Geometry check sheet. Reference: drawing and pictorial views, mm from the part's lowest x, y, z. Give positions to 0.01 mm unless a question says otherwise; leave off trailing zeros. Write each loop counter-clockwise with the first axis right and the second up, starting at its lowest first coordinate (ties: lowest second). Pieces come first, ordered by that corner, then holes.
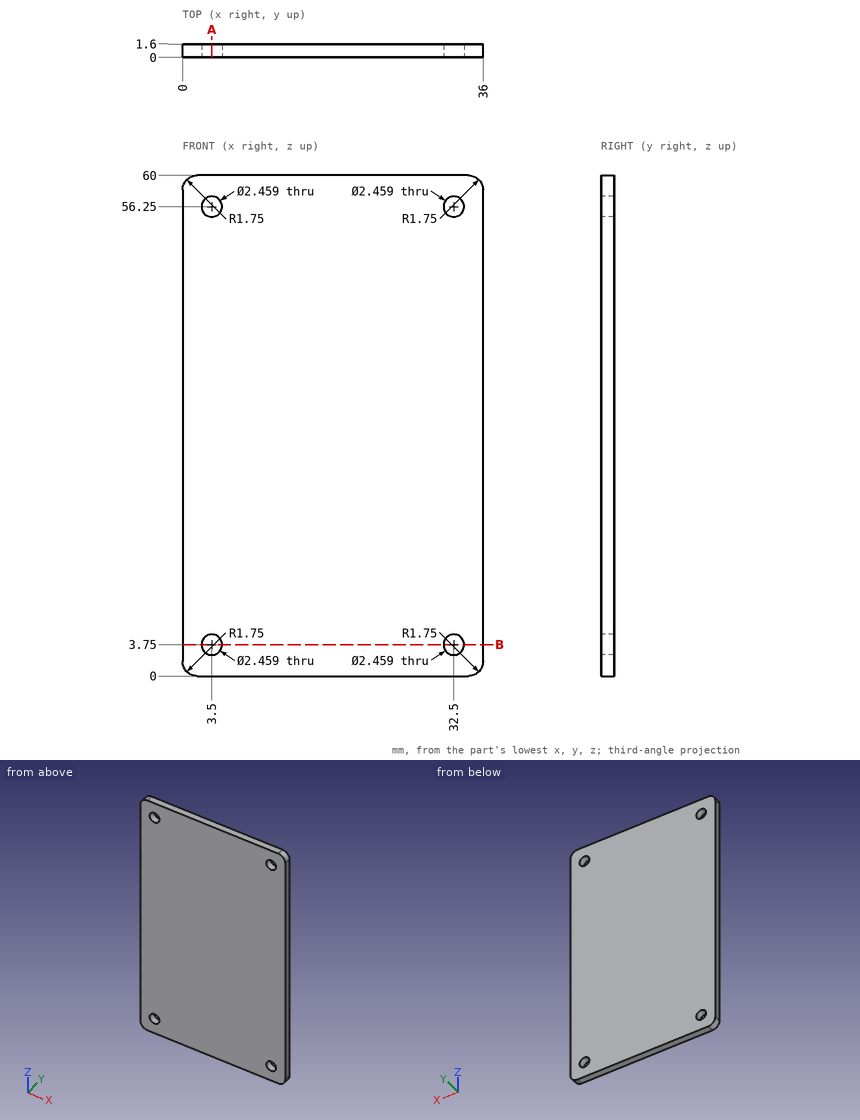
Item 1: Scan lines: line 1 along Z through (x, y) = (32.5, 1.2); line 2 along X through (y, z) = (0.3, 3.75). Record each from-to range of solid material in increasing order.
Answer key:
line 1: z = 0 to 2.52, 4.98 to 55.02, 57.48 to 60
line 2: x = 0 to 2.27, 4.73 to 31.27, 33.73 to 36
Item 2: Sectioned sample at A-A on x = 3.5. Record the cut outline in (y, z), then the cut area to 3 significant figures.
Answer key:
outline: (0, 0) - (1.6, 0) - (1.6, 2.52) - (0, 2.52) - close; (0, 4.98) - (1.6, 4.98) - (1.6, 55.02) - (0, 55.02) - close; (0, 57.48) - (1.6, 57.48) - (1.6, 60) - (0, 60) - close
area: 88.1 mm2
Item 3: Sectioned sample at B-B on z = 3.75. Record the cut outline in (x, y).
Answer key:
outline: (0, 0) - (2.27, 0) - (2.27, 1.6) - (0, 1.6) - close; (4.73, 0) - (31.27, 0) - (31.27, 1.6) - (4.73, 1.6) - close; (33.73, 0) - (36, 0) - (36, 1.6) - (33.73, 1.6) - close
Item 4: Depth check by flat-ended pin: pin 1 (2 mm diameter, centred on x = 32.5, z = 56.25, fed in from +Y). Enter the tip coordinate at first touch or a pass-through.
Answer key:
pin 1: passes through
